Here's how the part is built. I have some questions about the finished solid (model axes, mm). Face numbers are marked on the shaded views. Round coordinates to 2 decimals unless told otherwise and drop trailing zeros. Write each loop counter-clockwise with the first axis right and the second up, starting at its lowest first coordinate (ties: lowest second). Pieces come first, ordered by that corner, then holes. Notation, with made-up numbers: (26.5, 10.25) - (43.5, 10.25) arc R12 cw to (43.5, 29.25) - close; hole circle Ø3 at (6, 9). An arc over 180 degrees is marked (long way). Write item = value, one per line. Start each with the question number.
Item 1: For P1, Ø2, axis at x = 20, z = 31, coming from the -Y side; P2, Ø1, axis at x = -13, y = -24.5, coming from the +Z side, each with a flat end and sliding along its axis, tell me the tip position at first contact or that it passes through.
Item 2: If we section it at B-B (z = 0): Please give me the cut outline in (x, y), and give its area (3 significant figures).
Item 3: If we section it at D-D (z = 26): Please give me the cut outline in (x, y).
Item 4: If we section it at A-A (x = 0): Please give me the cut outline in (y, z).
Item 5: If I drill on line 1 along Z through (x, y) = (0, 21); line 2 along Z through (x, y) = (0, -9); line 3 along Y through (x, z) = (-42, -39), over which ranges is the centre line in solid material (lowest first)? Write a range as [from, to].
Item 6: If we section it at C-C (y = 14.5): Please give me the cut outline in (x, z).
Item 7: Thinking about a two-plate mould opening in X: for the marked faces 1, 2 and 3, which applies, pulls with the +X half, pulls with the -X half, needs draft (parallel to the pull), parting line crosses it, or undercut?
```python
from build123d import *

# Parameters (mm, degrees)
F0_R     = 22.799562
F0_R_2   = 13.477557
F1_DEPTH = 50.8
F2_DEPTH = 38.1


with BuildPart() as f1:
    # F0 (on Front) → F1 (new body)
    with BuildSketch(Plane.XZ):
        Polygon((53.325333, 44.9339), (0, 44.9339), (-53.325333, 44.9339), (-53.325333, 0), (-53.325333, -44.9339), (0, -44.9339), (53.325333, -44.9339), (53.325333, 0), align=None)
        Circle(F0_R, mode=Mode.SUBTRACT)
        Circle(F0_R)
        Circle(F0_R_2, mode=Mode.SUBTRACT)
    extrude(amount=-F1_DEPTH)

    # F0 (on Front) → F2 (join)
    with BuildSketch(Plane.XZ):
        Circle(F0_R)
        Circle(F0_R_2, mode=Mode.SUBTRACT)
    extrude(amount=F2_DEPTH)


solid = f1.part
```
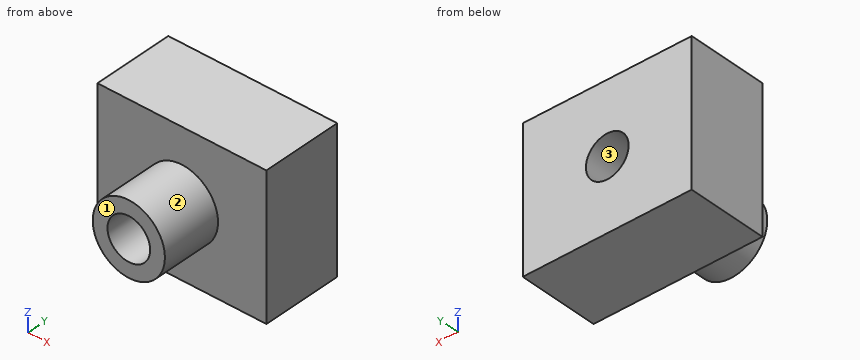
Reply:
q1.P1 = 0
q1.P2 = 19.07
q2.outline = (-53.33, 0) - (-22.8, 0) - (-22.8, -38.1) - (-13.48, -38.1) - (-13.48, 50.8) - (-53.33, 50.8) - close; (13.48, -38.1) - (22.8, -38.1) - (22.8, 0) - (53.33, 0) - (53.33, 50.8) - (13.48, 50.8) - close
q2.area = 4,760 mm2
q3.outline = (-53.33, 0) - (53.33, 0) - (53.33, 50.8) - (-53.33, 50.8) - close
q4.outline = (-38.1, -22.8) - (0, -22.8) - (0, -44.93) - (50.8, -44.93) - (50.8, -13.48) - (-38.1, -13.48) - close; (-38.1, 13.48) - (50.8, 13.48) - (50.8, 44.93) - (0, 44.93) - (0, 22.8) - (-38.1, 22.8) - close
q5.line_1 = [-44.93, -13.48], [13.48, 44.93]
q5.line_2 = [-22.8, -13.48], [13.48, 22.8]
q5.line_3 = [0, 50.8]
q6.outline = (-53.33, -44.93) - (53.33, -44.93) - (53.33, 44.93) - (-53.33, 44.93) - close; hole circle Ø26.96 at (0, 0)
q7.face_1 = needs draft
q7.face_2 = parting line crosses it
q7.face_3 = undercut
